Could you check a few things on this model? Use its own coordinates, in mm. Face numbers are marked on the shaded views. A direction names the side the tool comes from. Coordinates: 2 decimals unless noted, no trailing zeros. Order: outer loops, then holes, each group sorted by start corner. A loop starts at its lowest first (then second) coordinate and runs counter-clockwise, first axis right, second up. Notation, with made-up numbers: M 18.25,-18.5 L 76.25,-18.5 A13 cw 76.25,5.5 Z; hole C 32.5,64.5 d9. An arc over 180 degrees is marked long. Put each result on its own line as item: value. Start each with the question number.
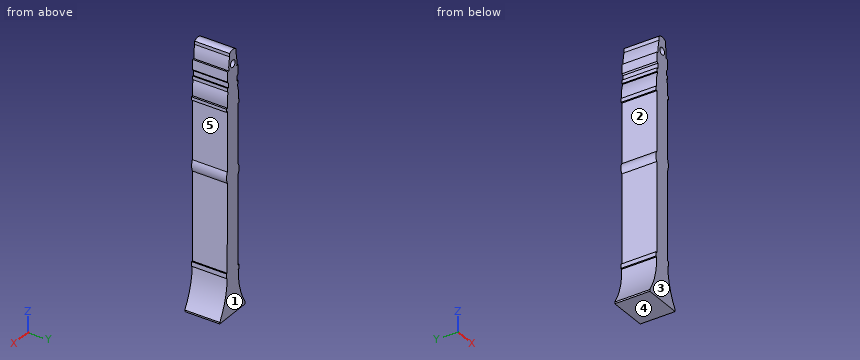
```python
from build123d import *

# Parameters (mm, degrees)
F1_DEPTH = 6.35
F2_R     = 0.644758
F3_DEPTH = 25.4


with BuildPart() as f1:
    # F0 (on Front) → F1 (new body)
    with BuildSketch(Plane.XZ):
        with BuildLine():
            Line((25.17445, 3.023418), (25.17445, 2.716777))
            Line((25.17445, 2.716777), (32.078393, 2.716777))
            Line((32.078393, 2.716777), (32.078393, 2.990841))
            ThreePointArc((32.078393, 2.990841), (30.603017, 6.307852), (30.058628, 9.897131))
            Line((30.058628, 9.897131), (30.28239, 9.87622))
            Line((30.28239, 9.87622), (30.281023, 10.708957))
            Line((30.281023, 10.708957), (30.058628, 10.708592))
            Line((30.058628, 10.708592), (30.032312, 26.736625))
            ThreePointArc((30.032312, 26.736625), (30.230598, 27.749797), (30.032312, 28.76297))
            Line((30.032312, 28.76297), (30.032312, 39.550062))
            Line((30.032312, 39.550062), (30.288203, 39.550062))
            Line((30.288203, 39.550062), (30.288203, 40.125817))
            Line((30.288203, 40.125817), (29.952377, 40.125817))
            ThreePointArc((29.952377, 40.125817), (30.032838, 41.588816), (29.772134, 43.030646))
            Line((29.772134, 43.030646), (29.952377, 43.030646))
            Line((29.952377, 43.030646), (29.952377, 43.664742))
            Line((29.952377, 43.664742), (29.76134, 43.664742))
            Line((29.76134, 43.664742), (29.76134, 44.51992))
            Line((29.76134, 44.51992), (29.992513, 44.805486))
            Line((29.992513, 44.805486), (29.944122, 46.605572))
            Line((29.944122, 46.605572), (29.634174, 46.605572))
            ThreePointArc((29.634174, 46.605572), (29.616481, 47.812826), (29.387884, 48.998371))
            Line((29.387884, 48.998371), (29.387884, 49.584199))
            ThreePointArc((29.387884, 49.584199), (28.53754, 49.887952), (27.687196, 49.584199))
            Line((27.687196, 49.584199), (27.687196, 48.860144))
            ThreePointArc((27.687196, 48.860144), (27.454964, 47.667764), (27.470311, 46.453077))
            Line((27.470311, 46.453077), (27.107688, 46.453077))
            Line((27.107688, 46.453077), (27.107688, 44.781074))
            Line((27.107688, 44.781074), (27.341686, 44.570461))
            Line((27.341686, 44.570461), (27.341686, 43.647271))
            Line((27.341686, 43.647271), (27.11089, 43.647271))
            Line((27.11089, 43.647271), (27.11089, 43.017823))
            Line((27.11089, 43.017823), (27.341686, 43.017823))
            ThreePointArc((27.341686, 43.017823), (27.001183, 41.641173), (27.039019, 40.223543))
            Line((27.039019, 40.223543), (26.824152, 40.223543))
            Line((26.824152, 40.223543), (26.824152, 39.525226))
            Line((26.824152, 39.525226), (27.076719, 39.525226))
            Line((27.076719, 39.525226), (27.076719, 28.713278))
            ThreePointArc((27.076719, 28.713278), (26.816318, 27.800124), (27.076719, 26.88697))
            Line((27.076719, 26.88697), (27.076719, 17.01922))
            Line((27.076719, 17.01922), (27.076719, 10.628499))
            Line((27.076719, 10.628499), (26.79955, 10.628499))
            Line((26.79955, 10.628499), (26.79955, 9.864554))
            Line((26.79955, 9.864554), (27.061559, 9.864554))
            ThreePointArc((27.061559, 9.864554), (26.613776, 6.307229), (25.17445, 3.023418))
        make_face()
    extrude(amount=F1_DEPTH)

    # F2 (on face) → F3 (cut)
    with BuildSketch(Plane.XZ.offset(6.35)):
        with Locations((28.552243, 47.344215)):
            Circle(F2_R)
    extrude(amount=-F3_DEPTH, mode=Mode.SUBTRACT)


solid = f1.part
```
Item 1: If we section it at B-B on z = 36.5: Write out the boundary of the cut face in (x, y), then the cut area to 3 significant figures.
Item 2: If we section it at A-A on x = 28.75: Write out the boundary of the cut face in (y, z).
Item 3: For pin 1 Ø3 at (x, y) = (30.5, -3) entering from +Z; pin 2 Ø1.8 at (y, z) = (-2, 45.5) entering from -X; pin 3 Ø0.6 at (y, z) = (-4.5, 40) entering from -X, each with a flat end and sliding along its axis, tell me the tip position at first contact or that it passes through.
Item 4: If we section it at C-C on z = 15: Write out the boundary of the cut face in (x, y).
Item 5: For the marked faces 1 and 2, which set-ups out of +Z, -Z, +X, -X, +Y, -Y let a thin tool reach every point of the face, with its end or its side?
Item 6: If we mould it in two halves opening along Z, with no side actions, what happens to the marked faces 3, 4 and 5? For each: released by +Z, released by -Z, zero draft, split by the parting line, or undercut.
Item 7: I need wall thicknesses on probe 1 along X at (y, z) = (-5.5, 33); probe 2 along X at (y, z) = (-1, 11); probe 3 along Z at (x, y) = (29, -3.25). Which ranges of each line are inside material? Lowest first, please.
Geometry check:
1. outline: M 27.08,-6.35 L 30.03,-6.35 L 30.03,0 L 27.08,0 Z
1. area: 18.8 mm²
2. outline: M -6.35,2.72 L 0,2.72 L 0,46.73 L -6.35,46.73 Z; M -6.35,47.96 L 0,47.96 L 0,49.87 L -6.35,49.87 Z
3. pin 1: stops at z = 49.81
3. pin 2: stops at x = 27.11
3. pin 3: stops at x = 26.82
4. outline: M 27.08,-6.35 L 30.05,-6.35 L 30.05,0 L 27.08,0 Z
5. face 1: +Z, -Z, +X, -X, +Y
5. face 2: -X, +Y, -Y
6. face 3: zero draft
6. face 4: released by -Z
6. face 5: undercut
7. probe 1: x = 27.08 to 30.03
7. probe 2: x = 27.08 to 30.06
7. probe 3: z = 2.72 to 46.88, 47.81 to 49.81
